Study the drawing (mm; zero at the part's minimum x, y, z) and answer. A direction names the side the tool comes from. Give positions to 0.01 mm unless a question says otherwise; leave off trailing zeros. Order: outer loops, then holes, each group sorted by start corner. A loop starts at its lowest first (then second) coordinate and runs counter-clockwise, first axis right, second up. Notation, with made-up numbers: (28.5, 21) -> (60.5, 21) arc R20 cw to (60.5, 40) -> close; hole circle Ø6 at (82.25, -39). An arc over 180 degrees is marked (long way). Use a Markdown table: item, result. Add a question column.
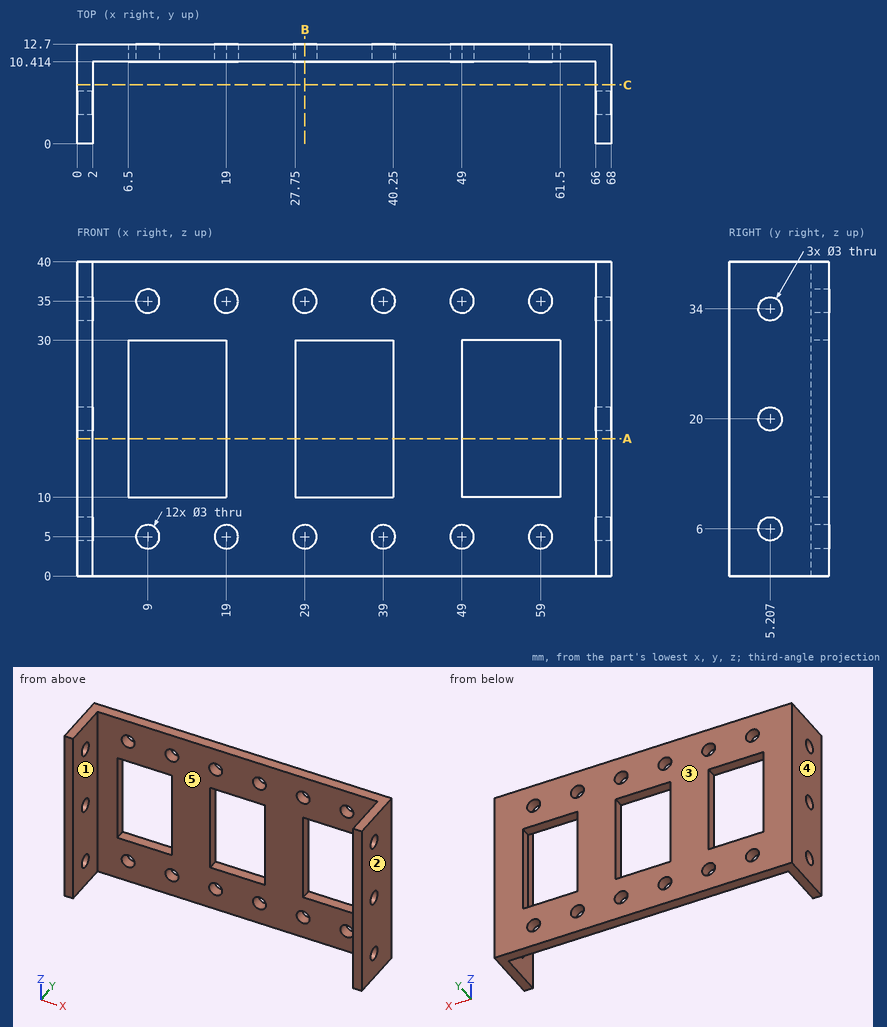
1) The part is cut by section A-A, the plane z = 17.5. Determine the outline of the cut face in (x, y), then the cut area to 3 significant figures.
2) Straight lines are drawn through the part: line 1 (Z direction, x = 9, y = 12.2); line 2 (X direction, y = 6.75, z = 37.5); line 3 (Y direction, x = 42, z = 35). For each, find the intervals that lie inside material, in ascending order.
3) A flat-ended cylindrical pin translates along its axis: pin 1 (4 mm diameter, centred on x = 39, z = 5, fed in from -Y). Find the tip coordinate at first contact, or state that the pin passes through.
4) Which of the six approach directions +Z, -Z, +X, -X, +Y, -Y give full straight-line access (tool end or side, diameter ignored) to the marked faces 1 and 2?
5) The part is cut by section C-C, the plane y = 7.5. Determine the outline of the cut face in (x, z).
6) The part is cut by section B-B, the plane x = 29. Determine the outline of the cut face in (y, z), then the cut area to 3 significant figures.
7) Determine the mould class of the marked faces 3, 4 and 5 for opening direction X: released by +X, released by -X, zero draft, split by the parting line, or undercut.
A:
| question | item | result |
|---|---|---|
| 1 | outline | (0, 0) -> (2, 0) -> (2, 10.41) -> (6.5, 10.41) -> (6.5, 12.7) -> (0, 12.7) -> close; (19, 10.41) -> (27.75, 10.41) -> (27.75, 12.7) -> (19, 12.7) -> close; (40.25, 10.41) -> (49, 10.41) -> (49, 12.7) -> (40.25, 12.7) -> close; (61.5, 10.41) -> (66, 10.41) -> (66, 0) -> (68, 0) -> (68, 12.7) -> (61.5, 12.7) -> close |
| 1 | area | 111 mm^2 |
| 2 | line 1 | 0 to 3.5, 6.5 to 10, 30 to 33.5, 36.5 to 40 |
| 2 | line 2 | 0 to 2, 66 to 68 |
| 2 | line 3 | 10.41 to 12.7 |
| 3 | pin 1 | y = 10.41 |
| 4 | face 1 | +Z, -Z, -Y |
| 4 | face 2 | +Z, -Z, +X, +Y, -Y |
| 5 | outline | (0, 0) -> (2, 0) -> (2, 40) -> (0, 40) -> close; (66, 0) -> (68, 0) -> (68, 40) -> (66, 40) -> close |
| 6 | outline | (10.41, 0) -> (12.7, 0) -> (12.7, 3.5) -> (10.41, 3.5) -> close; (10.41, 6.5) -> (12.7, 6.5) -> (12.7, 10) -> (10.41, 10) -> close; (10.41, 30) -> (12.7, 30) -> (12.7, 33.5) -> (10.41, 33.5) -> close; (10.41, 36.5) -> (12.7, 36.5) -> (12.7, 40) -> (10.41, 40) -> close |
| 6 | area | 32.0 mm^2 |
| 7 | face 3 | zero draft |
| 7 | face 4 | released by -X |
| 7 | face 5 | undercut |
